```python
from build123d import *

# Parameters (mm, degrees)
F0_R     = 27.1297247918
F1_DEPTH = 25.4
F2_R     = 19.1590274532
F3_DEPTH = 25.4
F4_R     = 11.5284679065
F5_DEPTH = 25.4
F6_R     = 6.766068174
F6_R_2   = 1.5282390362
F7_DEPTH = 25.4


# Not quite as in the source:
# - the program builds the solid bodies; features that only make, move or delete a surface that nothing else refers to are left out


with BuildPart() as f1:
    # F0 (on Front) → F1 (new body)
    with BuildSketch(Plane.XZ):
        Circle(F0_R)
    extrude(amount=F1_DEPTH)

    # F2 (on face) → F3 (join)
    with BuildSketch(Plane.XZ.offset(25.4)):
        Circle(F2_R)
    extrude(amount=F3_DEPTH)

    # F4 (on face) → F5 (join)
    with BuildSketch(Plane.XZ.offset(50.8)):
        Circle(F4_R)
    extrude(amount=F5_DEPTH)

    # F6 (on face) → F7 (join)
    with BuildSketch(Plane.XZ.offset(76.2)):
        Circle(F6_R)
        Circle(F6_R_2, mode=Mode.SUBTRACT)
    extrude(amount=F7_DEPTH)


solid = f1.part
```
Check sheet for the modelled part. Datum: model origin and axes. Units: mm. A direction names the side the tool comes from. Coordinates: 2 decimals unless noted, no trailing zeros. Loops run counter-clockwise (first coordinate to the right, second up) from the corner with the lowest first, then second, coordinate; pieces in that order, holes last.
1) Sectioned sample at D-D (y = -87). Record the boundary of the cut face in (x, z).
2) Release check for a two-part mould opening along Z. For faces 3 (the face through (-1.213, -88.722, -0.93)), 4 (the face through (-1.467, -88.722, -6.605)), 5 (the face through (0, -101.6, 2)) record: released by +Z, released by -Z, zero draft, split by the parting line, or undercut.
3) Sectioned sample at B-B (x = 0). Record the boundary of the cut face in (y, z).
4) Sectioned sample at A-A (z = 0). Record the boundary of the cut face in (x, y).
5) Access from +Z, -Z, +X, -X, +Y, -Y to the whole of each face (thin tool, end or side, straight path). Record for faces 1 (the face through (-4.153, -37.922, -18.703)), 2 (the face through (-27.103, -12.522, 1.193)).
6) Material ranges on probe 1 along Z at (x, y) = (0, -87.25); probe 2 along Y at (x, z) = (-20, -9); probe 3 along Y at (x, z) = (-10, 16), recorded low to high.
7) Sectioned sample at C-C (y = -62.5). Record the boundary of the cut face in (x, z).
8) Gauge pin test, flat ends, axial feed: pin 1 (8 mm diameter, centred on y = -54.5, z = 14, fed in from -X); pin 2 (1.5 mm diameter, centred on y = -60, z = -10.5, fed in from -X); pin 3 (3 mm diameter, centred on x = 15.5, z = 0, fed in from -Y). Record the tip position at first contact, or that the pin passes through.
Check sheet entries:
1. outline: circle Ø13.53 at (0, 0); hole circle Ø3.06 at (0, 0)
2. face 3: undercut
2. face 4: split by the parting line
2. face 5: zero draft
3. outline: (-101.6, -6.77) - (-76.2, -6.77) - (-76.2, -11.53) - (-50.8, -11.53) - (-50.8, -19.16) - (-25.4, -19.16) - (-25.4, -27.13) - (0, -27.13) - (0, 27.13) - (-25.4, 27.13) - (-25.4, 19.16) - (-50.8, 19.16) - (-50.8, 11.53) - (-76.2, 11.53) - (-76.2, 6.77) - (-101.6, 6.77) - (-101.6, 1.53) - (-76.2, 1.53) - (-76.2, -1.53) - (-101.6, -1.53) - close
4. outline: (-27.13, -25.4) - (-19.16, -25.4) - (-19.16, -50.8) - (-11.53, -50.8) - (-11.53, -76.2) - (-6.77, -76.2) - (-6.77, -101.6) - (-1.53, -101.6) - (-1.53, -76.2) - (1.53, -76.2) - (1.53, -101.6) - (6.77, -101.6) - (6.77, -76.2) - (11.53, -76.2) - (11.53, -50.8) - (19.16, -50.8) - (19.16, -25.4) - (27.13, -25.4) - (27.13, 0) - (-27.13, 0) - close
5. face 1: -Y
5. face 2: +Y, -Y
6. probe 1: z = -6.77 to -1.53, 1.53 to 6.77
6. probe 2: y = -25.4 to 0
6. probe 3: y = -50.8 to 0
7. outline: circle Ø23.06 at (0, 0)
8. pin 1: stops at x = -14.54
8. pin 2: stops at x = -6.15
8. pin 3: stops at y = -50.8
